Design review of the part built by this model. Coordinates are the model's own, in mm. Face numbers are marked on the shaded views. Coordinates: 2 decimals unless noted, no trailing zeros. Loops run counter-clockwise (first coordinate to the right, second up) from the corner with the lowest first, then second, coordinate; pieces in that order, holes last. Notation, with made-up numbers: (73, 2.5) -> (85, 2.5) arc R13 ccw to (85, 12.5) -> close; hole circle Ø8 at (64, 71.5). An arc over 180 degrees is marked (long way). One line per item, written item: value. Start each with the question number.
1. For probe 1 along Y at (x, z) = (2, 11.5); probe 2 along X at (y, z) = (29.1, 3.25); probe 3 along Y at (x, z) = (2.2, 0.75), list the stretches that pass through material, from the lowest coordinate up.
2. Draft analysis for pull direction X (two halves, no side actions). For the marked faces 1, 2 and 3, state which applies: pulls with the +X half, pulls with the -X half, needs draft (parallel to the pull), parting line crosses it, or undercut.
3. Add section A-A on x = -12.5. Write out the cut boundary in (y, z).
4. Add section C-C on z = -4. Write out the cut boundary in (x, y), plus the area to 3 significant figures.
5. Add section B-B on y = 19. Write out the cut boundary in (x, z).
6. Insertion check: pin 1 (6 mm diameter, centred on x = 0, y = 31.5, fed in from -Z); pin 2 (12 mm diameter, centred on x = 4, z = 0.5, fed in from +Y); pin 3 (3 mm diameter, centred on x = -30.5, y = 27.5, fed in from -Z); pin 4 (3 mm diameter, centred on x = 9, y = 34, fed in from +Z). Each pin has a flat end and moves straight along its axis. Give the tip position at first contact, or say it passes through.
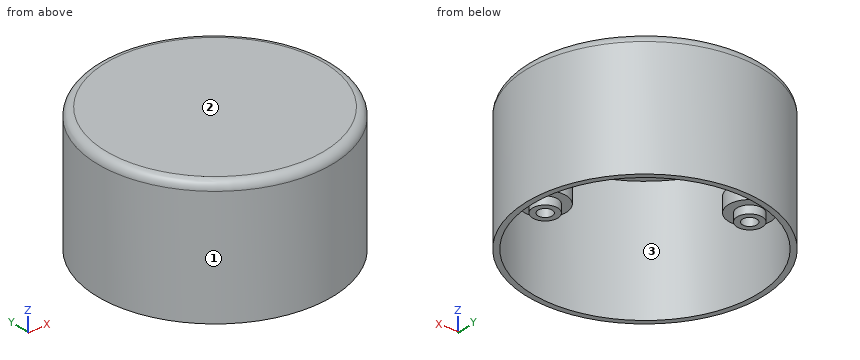
```python
from build123d import *

# Parameters (mm, degrees)
CYLINDER033_R     = 1.7
CYLINDER033_DEPTH = 8.5
CYLINDER036_R     = 5
CYLINDER036_DEPTH = 5.5
CHAMFER008_SIZE   = 2
CYLINDER031_R     = 3
CYLINDER031_DEPTH = 22.5
CYLINDER034_R     = 1.7
CYLINDER034_DEPTH = 8.5
CYLINDER035_R     = 5
CYLINDER035_DEPTH = 5.5
CHAMFER009_SIZE   = 2
CYLINDER032_R     = 3
CYLINDER032_DEPTH = 22.5
CYLINDER029_R     = 26.7
CYLINDER029_DEPTH = 30
CYLINDER030_R     = 28
CYLINDER030_DEPTH = 30
FILLET002_R       = 2
CHAMFER010_SIZE   = 1


with BuildPart() as obj1:
    # Cylinder033 → Cylinder033 (new body)
    with BuildSketch(Plane(origin=(2.2, 8, -3.4), x_dir=(1, 0, 0), z_dir=(0, 0, 1))):
        Circle(CYLINDER033_R)
    extrude(amount=CYLINDER033_DEPTH)


with BuildPart() as chamfer008:
    # Cylinder036 → Cylinder036 (new body)
    with BuildSketch(Plane(origin=(2.2, 8, -0.9), x_dir=(1, 0, 0), z_dir=(0, 0, 1))):
        Circle(CYLINDER036_R)
    extrude(amount=CYLINDER036_DEPTH)

    # Chamfer008
    chamfer008_edges = [chamfer008.edges().sort_by_distance(p)[0] for p in [
        (-2.8, 8, 4.6),
    ]]
    chamfer(chamfer008_edges, length=CHAMFER008_SIZE)


with BuildPart() as obj2:
    # Cylinder031 → Cylinder031 (new body)
    with BuildSketch(Plane(origin=(2.2, 8, -2.8), x_dir=(1, 0, 0), z_dir=(0, 0, 1))):
        Circle(CYLINDER031_R)
    extrude(amount=CYLINDER031_DEPTH)

    # Fusion003: union Chamfer008
    add(chamfer008.part)

    # Cut017: cut obj1
    add(obj1.part, mode=Mode.SUBTRACT)


with BuildPart() as obj3:
    # Cylinder034 → Cylinder034 (new body)
    with BuildSketch(Plane(origin=(-29.1, 29.1, -3.4), x_dir=(1, 0, 0), z_dir=(0, 0, 1))):
        Circle(CYLINDER034_R)
    extrude(amount=CYLINDER034_DEPTH)


with BuildPart() as chamfer009:
    # Cylinder035 → Cylinder035 (new body)
    with BuildSketch(Plane(origin=(-29.1, 29.1, -0.9), x_dir=(1, 0, 0), z_dir=(0, 0, 1))):
        Circle(CYLINDER035_R)
    extrude(amount=CYLINDER035_DEPTH)

    # Chamfer009
    chamfer009_edges = [chamfer009.edges().sort_by_distance(p)[0] for p in [
        (-34.1, 29.1, 4.6),
    ]]
    chamfer(chamfer009_edges, length=CHAMFER009_SIZE)


with BuildPart() as obj4:
    # Cylinder032 → Cylinder032 (new body)
    with BuildSketch(Plane(origin=(-29.1, 29.1, -2.8), x_dir=(1, 0, 0), z_dir=(0, 0, 1))):
        Circle(CYLINDER032_R)
    extrude(amount=CYLINDER032_DEPTH)

    # Fusion004: union Chamfer009
    add(chamfer009.part)

    # Cut018: cut obj3
    add(obj3.part, mode=Mode.SUBTRACT)


with BuildPart() as base_exterior_vaciado002:
    # Cylinder029 → Cylinder029 (new body)
    with BuildSketch(Plane(origin=(-12.5, 19, -10.6), x_dir=(1, 0, 0), z_dir=(0, 0, 1))):
        Circle(CYLINDER029_R)
    extrude(amount=CYLINDER029_DEPTH)


with BuildPart() as obj5:
    # Cylinder030 → Cylinder030 (new body)
    with BuildSketch(Plane(origin=(-12.5, 19, -10), x_dir=(1, 0, 0), z_dir=(0, 0, 1))):
        Circle(CYLINDER030_R)
    extrude(amount=CYLINDER030_DEPTH)

    # Cut016: cut base exterior vaciado002
    add(base_exterior_vaciado002.part, mode=Mode.SUBTRACT)

    # Fillet002
    fillet002_edges = [obj5.edges().sort_by_distance(p)[0] for p in [
        (-40.5, 19, 20),
    ]]
    fillet(fillet002_edges, radius=FILLET002_R)

    # Fusion005: union obj2, obj4
    add(obj2.part)
    add(obj4.part)

    # Chamfer010
    chamfer010_edges = [obj5.edges().sort_by_distance(p)[0] for p in [
        (-0.8, 8, 19.4),
        (-32.1, 29.1, 19.4),
    ]]
    chamfer(chamfer010_edges, length=CHAMFER010_SIZE)


solid = obj5.part
```
Worked answers:
1. probe 1: y = -4.95 to -3.42, 5.01 to 10.99, 41.42 to 42.95
1. probe 2: x = -38.61 to -37.22, -33.45 to -30.8, -27.4 to -24.75, 12.22 to 13.61
1. probe 3: y = -4.83 to -3.29, 3 to 6.3, 9.7 to 13, 41.29 to 42.83
2. face 1: parting line crosses it
2. face 2: needs draft
2. face 3: undercut
3. outline: (-9, -10) -> (-7.7, -10) -> (-7.7, 19.4) -> (45.7, 19.4) -> (45.7, -10) -> (47, -10) -> (47, 18) arc R2 ccw to (45, 20) -> (-7, 20) arc R2 ccw to (-9, 18) -> close
4. outline: circle Ø56 at (-12.5, 19); hole circle Ø53.4 at (-12.5, 19)
4. area: 223 mm²
5. outline: (-40.5, -10) -> (-39.2, -10) -> (-39.2, 19.4) -> (14.2, 19.4) -> (14.2, -10) -> (15.5, -10) -> (15.5, 18) arc R2 ccw to (13.5, 20) -> (-38.5, 20) arc R2 ccw to (-40.5, 18) -> close
6. pin 1: stops at z = 19.4
6. pin 2: stops at y = 44.96
6. pin 3: stops at z = -2.8
6. pin 4: stops at z = 20
